Part model, mm, in its own coordinate system. A direction names the side the tool comes from. Round coordinates to 2 decimals unless told otherwise and drop trailing zeros. Order: outer loops, then holes, each group sorted by start corner. A loop starts at its lowest first (then second) coordinate and runs counter-clockwise, first axis right, second up. Notation, with made-up numbers: (-4.75, 54) - (22.25, 54) arc R12 ccw to (22.25, 68) - close; hole circle Ø2 at (78, 60.25). An arc over 180 degrees is marked (long way). Return JSON: item names as keys, results as strings. Group by question number.
Item 1: Saw through at D-D on x = 6. List the corners of the cut face in (y, z).
Item 2: Probe probe 1 along Z at (x, y) = (0, -10.5); probe 2 along X at (y, z) = (-1.5, 17); probe 3 along Z at (x, y) = (0, -5). List the from-to ranges inside material, lowest first.
Item 3: Drop flat-ended pins along their axis: pin 1 (5 mm diameter, centred on y = -10, z = 14.5, fed in from -X); pin 2 (1.5 mm diameter, centred on x = -1, z = 7, fed in from +Y); pin 3 (2.5 mm diameter, centred on x = -1, y = 0, fed in from +Z); pin 4 (3 mm diameter, centred on x = 0, z = 28.5, fed in from +Y). Give the stop position or say it passes through.
Item 4: Two-plate mould, pull along Y, no slides. Class faces 4 (the face through (12.932, -5.362, 16.269)), 5 (the face through (-6.5, 0, 29)), 6 (the face through (3.43, 0.07, -6)): released by +Y, released by -Y, zero draft, split by the parting line, or undercut.
Item 5: Saw through at B-B on y = 6.75. List the corners of the cut face in (x, z), and give its area (3 significant figures).
Item 6: Saw through at C-C on z = 29.5. List the corners of the cut face in (x, y), and give its area (3 significant figures).
Item 7: Saw through at A-A on z = 1. List the corners of the cut face in (x, y), and give its area (3 significant figures).
Item 8: Tool access for faces 1 (the face through (0, 1.5, 31)), 2 (the face through (5, 1.6, 8.7)), 3 (the face through (0, -3, 33)): list every direction of +Z, -Z, +X, -X, +Y, -Y with a clear straight run to the whole face (end or side of a thin tool).
```python
from build123d import *

# Parameters (mm, degrees)
F0_R      = 14
F0_R_2    = 13
F0_R_3    = 5.25
F1_DEPTH  = 33
F2_DEPTH  = 6
F3_R      = 14
F3_R_2    = 5.25
F4_DEPTH  = 10
F7_W      = 13
F7_H      = 3
F8_DEPTH  = 9
F9_R      = 2
F10_DEPTH = 16


with BuildPart() as f1:
    # F0 (on Top) → F1 (new body)
    with BuildSketch(Plane.XY):
        Circle(F0_R)
        Circle(F0_R_2, mode=Mode.SUBTRACT)
        Circle(F0_R_3)
        Polygon((-3.229793, 1.910961), (0.040044, 3.752563), (3.269837, 1.841602), (3.229793, -1.910961), (-0.040044, -3.752563), (-3.269837, -1.841602), align=None, mode=Mode.SUBTRACT)
    extrude(amount=F1_DEPTH)

    # F0 (on Top) → F2 (join)
    with BuildSketch(Plane.XY):
        Circle(F0_R_3)
        Polygon((-3.229793, 1.910961), (0.040044, 3.752563), (3.269837, 1.841602), (3.229793, -1.910961), (-0.040044, -3.752563), (-3.269837, -1.841602), align=None, mode=Mode.SUBTRACT)
    extrude(amount=-F2_DEPTH)


with BuildPart() as f4:
    # F3 (on face) → F4 (new body)
    with BuildSketch(Plane.XY.offset(33)):
        Circle(F3_R)
        Circle(F3_R_2, mode=Mode.SUBTRACT)
        Polygon((-3.229793, 1.910961), (-3.269837, -1.841602), (-0.040044, -3.752563), (3.229793, -1.910961), (3.269837, 1.841602), (0.040044, 3.752563), align=None)
    extrude(amount=-F4_DEPTH)


with BuildPart() as f1_1:
    add(f1.part)

    # F5: union F4
    add(f4.part)

    # F6: union 

    # F7 (on face) → F8 (cut)
    with BuildSketch(Plane.XY.offset(33)):
        Rectangle(F7_W, F7_H)
    extrude(amount=-F8_DEPTH, mode=Mode.SUBTRACT)

    # F9 (on face) → F10 (cut, symmetric)
    with BuildSketch(Plane.XZ.offset(-1.5)):
        with Locations((0, 28.5)):
            Circle(F9_R)
    extrude(amount=F10_DEPTH, both=True, mode=Mode.SUBTRACT)


solid = f1_1.part
```
Filled in:
{
 "1": {"outline": "(-12.65, 0) - (-11.53, 0) - (-11.53, 23) - (11.53, 23) - (11.53, 0) - (12.65, 0) - (12.65, 33) - (1.5, 33) - (1.5, 24) - (-1.5, 24) - (-1.5, 33) - (-12.65, 33) - close"},
 "2": {"probe 1": "z = 23 to 26.5, 30.5 to 33", "probe 2": "x = -13.92 to -12.91, -5.03 to -3.27, 3.23 to 5.03, 12.91 to 13.92", "probe 3": "z = -6 to 26.5, 30.5 to 33"},
 "3": {"pin 1": "stops at x = -11.82", "pin 2": "stops at y = 14", "pin 3": "stops at z = 24", "pin 4": "passes through"},
 "4": {"face 4": "split by the parting line", "face 5": "undercut", "face 6": "zero draft"},
 "5": {"outline": "(-12.27, 0) - (-11.11, 0) - (-11.11, 23) - (11.11, 23) - (11.11, 0) - (12.27, 0) - (12.27, 33) - (-12.27, 33) - close; hole circle Ø4 at (0, 28.5)", "area": "286 mm^2"},
 "6": {"outline": "(-6.5, -1.5) - (-6.5, 1.5) - (-1.73, 1.5) - (-1.73, 13.89) arc R14 ccw to (-1.73, -13.89) - (-1.73, -1.5) - close; (1.73, -13.89) arc R14 ccw to (1.73, 13.89) - (1.73, 1.5) - (6.5, 1.5) - (6.5, -1.5) - (1.73, -1.5) - close", "area": "490 mm^2"},
 "7": {"outline": "circle Ø28 at (0, 0); circle Ø10.5 at (0, 0); hole circle Ø26 at (0, 0); hole (-3.27, -1.84) - (-0.04, -3.75) - (3.23, -1.91) - (3.27, 1.84) - (0.04, 3.75) - (-3.23, 1.91) - close", "area": "135 mm^2"},
 "8": {"face 1": "+Z", "face 2": "-Z", "face 3": "+Z, +X, -X, +Y, -Y"}
}
